Part model, mm, in its own coordinate system. A direction names the side the tool comes from. Round coordinates to 2 decimals unless told otherwise and drop trailing zeros. Loops run counter-clockwise (first coordinate to the right, second up) from the corner with the lowest first, then second, coordinate; pieces in that order, holes last.
1) Band-saw the part on B-B, the plane z = -98.5. Write the cut outline in (x, y), then the cut area to 4 significant figures.
2) 3-axis set-ups, long thin cutter, end or side, ignore diameter. For faces 1 (the flat face through (1.479, 67.635, 29.269)), 2 (the flat face through (1.479, 65.594, -52.364)): which of +Z, -Z, +X, -X, +Y, -Y reach the whole face in a straight line?
3) Band-saw the part on D-D, the plane x = 0.5. State how many separate pieces and enclosed holes the cut face has, then the cut area to 3 significant figures.
4) Band-saw the part on A-A, the plane y = 104.5. Write the cut outline in (x, z).
5) Drop flat-ended pins along their axis: P1, Ø1.5, axis at x = 2, y = -28.5, coming from the -Z side; P2, Ø1.5, axis at x = 2, y = 33, coming from the +Z side; P3, Ø1.5, axis at x = 2, y = 31, coming from the -Z side. Give the stop position or say it passes through.
6) Mould opens along Z. For faces 3 (the flat face through (3, 31, 23)), 4 (the flat face through (1.479, 107.901, 68.946)), 5 (the flat face through (1.479, 43.849, -32.044)) say: +Z half, -Z half, draft (parallel to the pull), parting line (faces both ways), or undercut.
7) Band-saw the part on C-C, the plane y = 177. Write the cut outline in (x, z), then the cut area to 3 significant figures.
8) Probe line 1 (Y direction, x = 1.5, z = 125.5); line 2 (Z direction, x = 0.6, y = 128); line 3 (Y direction, x = 2.9, z = 119). List the from-to ranges inside material, lowest first.
from build123d import *

# Parameters (mm, degrees)
BOSS_EXTRUDE1_DEPTH     = 3
SKETCH2_W               = 27.727272727
SKETCH2_H               = 3
SKETCH2_W_2             = 3
SKETCH2_H_2             = 18
SKETCH2_H_3             = 9
SKETCH2_W_3             = 23.343342349
SKETCH2_W_4             = 23.34334235
SKETCH2_W_5             = 6
CUT_EXTRUDE1_DEPTH      = 1
CUT_EXTRUDE1_DEPTH_BACK = 4
SKETCH3_W               = 3.2
SKETCH3_H               = 10.5
SKETCH3_W_2             = 5.2
SKETCH3_H_2             = 2.5
CUT_EXTRUDE2_DEPTH      = 1
CUT_EXTRUDE2_DEPTH_BACK = 4
FILLET1_R               = 2.5
BOSS_EXTRUDE2_DEPTH     = 3
FILLET2_R               = 2.5
SKETCH6_R               = 5
SKETCH6_R_2             = 1.65
CUT_EXTRUDE5_DEPTH      = 1
CUT_EXTRUDE5_DEPTH_BACK = 4
SKETCH8_R               = 10
SKETCH8_W               = 5
SKETCH8_H               = 1
CUT_EXTRUDE6_DEPTH      = 4
CUT_EXTRUDE6_DEPTH_BACK = 1
SKETCH8_4_R             = 10
SKETCH8_4_W             = 5
SKETCH8_4_H             = 1
BOSS_EXTRUDE4_DEPTH     = 3
SKETCH9_W               = 20
SKETCH9_H               = 3
CUT_EXTRUDE7_DEPTH      = 4
CUT_EXTRUDE7_DEPTH_BACK = 1
SKETCH10_W              = 27.840909091
SKETCH10_H              = 3
CUT_EXTRUDE8_DEPTH      = 4
CUT_EXTRUDE8_DEPTH_BACK = 1


with BuildPart() as part:
    # Sketch1 → Boss-Extrude1 (new body)
    with BuildSketch(Plane(origin=(0, 0, 0), x_dir=(0, 0, -1), z_dir=(1, 0, 0))):
        with BuildLine():
            Line((-152.5, 33), (152.5, 33))
            Line((152.5, 33), (152.5, 23))
            Line((152.5, 23), (107.5, 23))
            ThreePointArc((107.5, 23), (72.144660941, 8.355339059), (57.5, -27))
            Line((57.5, -27), (57.5, -33))
            Line((57.5, -33), (-152.5, -33))
            Line((-152.5, -33), (-152.5, 33))
        make_face()
    extrude(amount=BOSS_EXTRUDE1_DEPTH)

    # Sketch2 → Cut-Extrude1 (cut, two sides)
    with BuildSketch(Plane(origin=(3, 0, 0), x_dir=(0, 0, -1), z_dir=(1, 0, 0))) as cut_extrude1_sk:
        with Locations((-138.636363636, 31.5)):
            Rectangle(SKETCH2_W, SKETCH2_H)
        with Locations((-83.181818182, 31.5)):
            Rectangle(SKETCH2_W, SKETCH2_H)
        with Locations((-27.727272728, 31.5)):
            Rectangle(SKETCH2_W, SKETCH2_H)
        with Locations((-151, 3)):
            Rectangle(SKETCH2_W_2, SKETCH2_H_2)
        with Locations((-151, -28.5)):
            Rectangle(SKETCH2_W_2, SKETCH2_H_3)
        with Locations((-117.484986475, -28.5)):
            Rectangle(SKETCH2_W_3, SKETCH2_H)
        with Locations((-70.798301777, -28.5)):
            Rectangle(SKETCH2_W_3, SKETCH2_H)
        with Locations((22.575067622, -28.5)):
            Rectangle(SKETCH2_W_4, SKETCH2_H)
        with Locations((149.5, 31.5)):
            Rectangle(SKETCH2_W_5, SKETCH2_H)
        with Locations((-24.111617078, -28.5)):
            Rectangle(SKETCH2_W_3, SKETCH2_H)
    extrude(amount=CUT_EXTRUDE1_DEPTH, mode=Mode.SUBTRACT)
    extrude(cut_extrude1_sk.sketch, amount=-CUT_EXTRUDE1_DEPTH_BACK, mode=Mode.SUBTRACT)

    # Sketch3 → Cut-Extrude2 (cut, two sides)
    with BuildSketch(Plane(origin=(3, 0, 0), x_dir=(0, 0, -1), z_dir=(1, 0, 0))) as cut_extrude2_sk:
        with Locations((-110.909090909, 27.75)):
            Rectangle(SKETCH3_W, SKETCH3_H)
        with Locations((-110.909090909, 28.575)):
            Rectangle(SKETCH3_W_2, SKETCH3_H_2)
    extrude(amount=CUT_EXTRUDE2_DEPTH, mode=Mode.SUBTRACT)
    extrude(cut_extrude2_sk.sketch, amount=-CUT_EXTRUDE2_DEPTH_BACK, mode=Mode.SUBTRACT)

    # Fillet1
    fillet1_edges = [part.edges().sort_by_distance(p)[0] for p in [
        (1.5, -33, -57.5),
    ]]
    fillet(fillet1_edges, radius=FILLET1_R)

    # Sketch4 → Boss-Extrude2 (add)
    with BuildSketch(Plane(origin=(0, 0, 0), x_dir=(0, 0, -1), z_dir=(1, 0, 0))):
        with BuildLine():
            Line((-83.181818182, 33), (-83.181818182, 30))
            Line((-83.181818182, 30), (35.818181818, 30))
            Line((35.818181818, 30), (35.818181818, 33))
            Line((35.818181818, 33), (25.753026775, 61.931534749))
            Line((25.753026775, 61.931534749), (59.886459158, 33))
            Line((59.886459158, 33), (90.818181818, 33))
            Line((90.818181818, 33), (12.817635516, 99.113348651))
            Line((12.817635516, 99.113348651), (-16.565017269, 183.571584658))
            ThreePointArc((-16.565017269, 183.571584658), (-36.922973482, 196.946020133), (-55.102803407, 180.73442893))
            Line((-55.102803407, 180.73442893), (-83.181818182, 33))
        make_face()
        Polygon((-54.643252411, 49.263022537), (-34.033564648, 157.698467174), (-8.047004759, 83.002045982), align=None, mode=Mode.SUBTRACT)
        Polygon((-3.929894771, 71.167721507), (6.913219914, 40), (-46.974972009, 40), align=None, mode=Mode.SUBTRACT)
    extrude(amount=BOSS_EXTRUDE2_DEPTH)

    # Fillet2
    fillet2_edges = [part.edges().sort_by_distance(p)[0] for p in [
        (1.5, 33, -59.886459158),
        (1.5, 61.931534749, -25.753026775),
        (1.5, 33, -35.818181818),
        (1.5, 40, -6.913219914),
        (1.5, 71.167721507, 3.929894771),
        (1.5, 40, 46.974972009),
        (1.5, 49.263022537, 54.643252411),
        (1.5, 83.002045982, 8.047004759),
        (1.5, 157.698467174, 34.033564648),
    ]]
    fillet(fillet2_edges, radius=FILLET2_R)

    # Sketch6 → Cut-Extrude5 (cut, two sides)
    with BuildSketch(Plane(origin=(3, 0, 0), x_dir=(0, 0, -1), z_dir=(1, 0, 0))) as cut_extrude5_sk:
        with Locations((-35.454545455, 177)):
            Circle(SKETCH6_R)
        with Locations((-1.492946709, 95.333591431)):
            Circle(SKETCH6_R_2)
        with Locations((27.342535354, 25.993797473)):
            Circle(SKETCH6_R_2)
    extrude(amount=CUT_EXTRUDE5_DEPTH, mode=Mode.SUBTRACT)
    extrude(cut_extrude5_sk.sketch, amount=-CUT_EXTRUDE5_DEPTH_BACK, mode=Mode.SUBTRACT)

    # Sketch8 → Cut-Extrude6 (cut, two sides)
    with BuildSketch(Plane(origin=(0, 0, 0), x_dir=(0, 0, -1), z_dir=(1, 0, 0))) as cut_extrude6_sk:
        with Locations((-40, 0)):
            Circle(SKETCH8_R)
        with Locations((-5, 0)):
            Rectangle(SKETCH8_W, SKETCH8_H)
    extrude(amount=CUT_EXTRUDE6_DEPTH, mode=Mode.SUBTRACT)
    extrude(cut_extrude6_sk.sketch, amount=-CUT_EXTRUDE6_DEPTH_BACK, mode=Mode.SUBTRACT)

    # Sketch8_4 → Boss-Extrude4 (add)
    with BuildSketch(Plane(origin=(0, 0, 0), x_dir=(0, 0, -1), z_dir=(1, 0, 0))):
        with Locations((-40, 0)):
            Circle(SKETCH8_4_R)
        with Locations((-5, 0)):
            Rectangle(SKETCH8_4_W, SKETCH8_4_H)
    extrude(amount=BOSS_EXTRUDE4_DEPTH)

    # Sketch9 → Cut-Extrude7 (cut, two sides)
    with BuildSketch(Plane(origin=(0, 0, 0), x_dir=(0, 0, -1), z_dir=(1, 0, 0))) as cut_extrude7_sk:
        Polygon((-68.111670983, 53.378521315), (-64.377242053, 73.026779267), (-61.43000336, 72.466614928), (-65.16443229, 52.818356975), align=None)
        Polygon((-55.507973344, 119.691391905), (-52.707151647, 134.427585369), (-49.759912954, 133.867421029), (-52.560734651, 119.131227565), align=None)
        Polygon((64.311409407, 40.391956194), (49.054577079, 53.32366402), (50.994333253, 55.612188869), (66.251165581, 42.680481043), align=None)
        with Locations((-17.931502251, 33)):
            Rectangle(SKETCH9_W, SKETCH9_H)
    extrude(amount=CUT_EXTRUDE7_DEPTH, mode=Mode.SUBTRACT)
    extrude(cut_extrude7_sk.sketch, amount=-CUT_EXTRUDE7_DEPTH_BACK, mode=Mode.SUBTRACT)

    # Sketch10 → Cut-Extrude8 (cut, two sides)
    with BuildSketch(Plane(origin=(0, 0, 0), x_dir=(0, 0, -1), z_dir=(1, 0, 0))) as cut_extrude8_sk:
        with Locations((104.738636364, 31.5)):
            Rectangle(SKETCH10_W, SKETCH10_H)
    extrude(amount=CUT_EXTRUDE8_DEPTH, mode=Mode.SUBTRACT)
    extrude(cut_extrude8_sk.sketch, amount=-CUT_EXTRUDE8_DEPTH_BACK, mode=Mode.SUBTRACT)


solid = part.part
Reported:
1. outline: (0, 22.18) - (3, 22.18) - (3, 30) - (0, 30) - close
1. area: 23.45 mm2
2. face 1: +X, -X
2. face 2: -Z, +X, -X, +Y
3. separate pieces: 1
3. enclosed holes: 14
3. area: 25,100 mm2
4. outline: (0, -10.94) - (3, -10.94) - (3, 15.53) - (0, 15.53) - close; (0, 44.14) - (3, 44.14) - (3, 69.59) - (0, 69.59) - close
5. P1: stops at z = -57.5
5. P2: stops at z = 124.77
5. P3: stops at z = -146.5
6. face 3: draft
6. face 4: +Z half
6. face 5: undercut
7. outline: (0, 14.28) - (3, 14.28) - (3, 30.45) - (0, 30.45) - close; (0, 40.45) - (3, 40.45) - (3, 55.81) - (0, 55.81) - close
7. area: 94.6 mm2
8. line 1: y = -33 to -30, -27 to 30
8. line 2: z = -2.77 to 23.7, 39.68 to 50.88, 53.93 to 65.13
8. line 3: y = -33 to -30, -27 to 33
